from build123d import *

# Parameters (mm, degrees)
F0_R        = 12.7
F1_DEPTH    = 88.9
F2_W        = 20
F2_H        = 10
F3_DEPTH    = 19.05
F4_T1_DEPTH = 45.4


# Not quite as in the source:
# - a fillet or chamfer that OpenCascade refuses, or shapes differently, is made with other operations: its cross-section is extruded or revolved along the edge and cut away or added


with BuildPart() as f1:
    # F0 (on Front) → F1 (new body)
    with BuildSketch(Plane.XZ):
        Circle(F0_R)
    extrude(amount=F1_DEPTH)

    # F2 (on face) → F3 (join)
    with BuildSketch(Plane.XZ.offset(88.9)):
        Rectangle(F2_W, F2_H)
    extrude(amount=F3_DEPTH)

    # F4: fillet of radius 5.08 on 2 edges, made by hand

    # F4_s2 → F4_t1 (cut)
    with BuildSketch(Plane.YZ.offset(-22.7)):
        with BuildLine():
            ThreePointArc((-102.87, 5), (-106.4621024484, 3.5121024484), (-107.95, -0.08))
            Line((-107.95, -0.08), (-107.95, 5))
            Line((-107.95, 5), (-102.87, 5))
        make_face()
        with BuildLine():
            ThreePointArc((-102.87, -5), (-106.4621024484, -3.5121024484), (-107.95, 0.08))
            Line((-107.95, 0.08), (-107.95, -5))
            Line((-107.95, -5), (-102.87, -5))
        make_face()
    extrude(amount=F4_T1_DEPTH, mode=Mode.SUBTRACT)


solid = f1.part
Verification items for the finished model (mm, model axes). A direction names the side the tool comes from. Coordinates: 2 decimals unless noted, no trailing zeros. Write each loop counter-clockwise with the first axis right and the second up, starting at its lowest first coordinate (ties: lowest second). Pieces come first, ordered by that corner, then holes. Notation, with made-up numbers: M 49.5,-33 L 104.5,-33 A25 cw 104.5,-5 Z; hole C 78.5,85 d3. An arc over 180 degrees is marked long. Use a Markdown table: item, result.
Q1. Sectioned sample at B-B, the plane z = -2. Record the boundary of the cut face in (x, y), plus the area to 3 significant figures.
Reply:
| item | result |
|---|---|
| outline | M -12.54,-88.9 L -10,-88.9 L -10,-107.5 L 10,-107.5 L 10,-88.9 L 12.54,-88.9 L 12.54,0 L -12.54,0 Z |
| area | 2,600 mm² |
Q2. Set-up check for faces 1 (the face through (0, -96, 5)), 2 (the face through (-10, -98, 0)), 3 (the face through (0, -96, -5)): record each of +Z, -Z, +X, -X, +Y, -Y from which the full face is reachable in a straight line by a thin tool's end or side.
Reply:
| item | result |
|---|---|
| face 1 | +Z, +X, -X, -Y |
| face 2 | +Z, -Z, -X, -Y |
| face 3 | -Z, +X, -X, -Y |
Q3. Sectioned sample at C-C, the plane y = -19. Record the boundary of the cut face in (x, z), plus the area to 3 significant figures.
Reply:
| item | result |
|---|---|
| outline | C 0,0 d25.4 |
| area | 507 mm² |
Q4. Sectioned sample at D-D, the plane z = 3.75. Record the boundary of the cut face in (x, y), plus the area to 3 significant figures.
Reply:
| item | result |
|---|---|
| outline | M -12.13,-88.9 L -10,-88.9 L -10,-106.21 L 10,-106.21 L 10,-88.9 L 12.13,-88.9 L 12.13,0 L -12.13,0 Z |
| area | 2,500 mm² |
Q5. Go/stop test with flat-tipped pins: P1, Ø8, axis at x = 7.5, y = -21.5, coming from the +Z side; P2, Ø7.5, axis at x = -3.5, z = -4.5, coming from the -Y side; P3, Ø11, axis at x = -4.5, y = -99, coming from the -Z side. Record where each tip stops, or that it passes through.
Reply:
| item | result |
|---|---|
| P1 | stops at z = 12.21 |
| P2 | stops at y = -107.88 |
| P3 | stops at z = -5 |
Q6. Thickness scan on line 1 (X direction, y = -5, z = -0.25); line 2 (Y direction, x = 5, z = -6.75); line 3 (Y direction, x = -3, z = 0.25). Record the ranges inside material, lowest first.
Reply:
| item | result |
|---|---|
| line 1 | x = -12.7 to 12.7 |
| line 2 | y = -88.9 to 0 |
| line 3 | y = -107.94 to 0 |
Q7. Sectioned sample at A-A, the plane x = 0. Record the boundary of the cut face in (y, z).
Reply:
| item | result |
|---|---|
| outline | M -107.95,0 A5.08 ccw -102.87,-5 L -88.9,-5 L -88.9,-12.7 L 0,-12.7 L 0,12.7 L -88.9,12.7 L -88.9,5 L -102.87,5 A5.08 ccw Z |
